from build123d import *

# Parameters (mm, degrees)
SKETCH1_R           = 3
SKETCH1_W           = 3.88
SKETCH1_H           = 3
BOSS_EXTRUDE1_DEPTH = 3
SKETCH2_R           = 1.0009
CUT_EXTRUDE1_DEPTH  = 516.692890771


with BuildPart() as part:
    # Sketch1 → Boss-Extrude1 (new body)
    with BuildSketch(Plane.XY):
        Polygon((-398.2841, 298.0765), (-386.271234014, 299.794262601), (-329.587365996, 299.794262601), (-329.587365996, 281.358737399), (-386.271234014, 281.358737399), (-398.2841, 283.0765), (-419.587365996, 283.0765), (-419.587365996, 298.0765), align=None)
        with Locations((-404.586054436, 290.5765)):
            Circle(SKETCH1_R, mode=Mode.SUBTRACT)
        with Locations((-369.044562351, 293.935134885)):
            Rectangle(SKETCH1_W, SKETCH1_H, mode=Mode.SUBTRACT)
        with Locations((-369.044562351, 285.640934885)):
            Rectangle(SKETCH1_W, SKETCH1_H, mode=Mode.SUBTRACT)
        with Locations((-341.542562351, 293.935134885)):
            Rectangle(SKETCH1_W, SKETCH1_H, mode=Mode.SUBTRACT)
        with Locations((-341.542562351, 285.640934885)):
            Rectangle(SKETCH1_W, SKETCH1_H, mode=Mode.SUBTRACT)
    extrude(amount=BOSS_EXTRUDE1_DEPTH)

    # Sketch2 → Cut-Extrude1 (cut, through all)
    with BuildSketch(Plane.XY.offset(3)):
        with Locations((-414.786054436, 290.5765)):
            Circle(SKETCH2_R)
        with Locations((-410.936054436, 290.5765)):
            Circle(SKETCH2_R)
        with Locations((-398.236054436, 290.5765)):
            Circle(SKETCH2_R)
        with Locations((-394.386054436, 290.5765)):
            Circle(SKETCH2_R)
    extrude(amount=-CUT_EXTRUDE1_DEPTH, mode=Mode.SUBTRACT)


solid = part.part
Design review of the part built by this model. Coordinates are the model's own, in mm. A direction names the side the tool comes from. Round coordinates to 2 decimals unless told otherwise and drop trailing zeros. Order: outer loops, then holes, each group sorted by start corner. A loop starts at its lowest first (then second) coordinate and runs counter-clockwise, first axis right, second up.
1) For L1, parallel to Y at x = -340.5, z = 2.4; L2, parallel to X at y = 290.5, z = 2.75; L3, parallel to X at y = 285.5, z = 0.7, list the stretches that pass through material, from the lowest coordinate up.
The answers:
L1: y = 281.36 to 284.14, 287.14 to 292.44, 295.44 to 299.79
L2: x = -419.59 to -415.78, -413.79 to -411.93, -409.94 to -407.59, -401.59 to -399.23, -397.24 to -395.38, -393.39 to -329.59
L3: x = -419.59 to -370.98, -367.1 to -343.48, -339.6 to -329.59
2) Draft analysis for pull direction X (two halves, no side actions). For faces 4 (the flat face through (-329.587, 291, 1)), 5 (the flat face through (-370.985, 294, 1)), 6 (the flat face through (-392.194, 282.206, 1.479)), 7 (the flat face through (-374, 291, 3)), state which applies: released by +X, released by -X, zero draft, split by the parting line, or undercut.
The answers:
face 4: released by +X
face 5: undercut
face 6: released by -X
face 7: zero draft
3) Consider section A-A (y = 286). State the section outline as (x, z) points.
The answers:
outline: (-419.59, 0) - (-370.98, 0) - (-370.98, 3) - (-419.59, 3) - close; (-367.1, 0) - (-343.48, 0) - (-343.48, 3) - (-367.1, 3) - close; (-339.6, 0) - (-329.59, 0) - (-329.59, 3) - (-339.6, 3) - close
4) Consider section B-B (z = 1.4). Count the separate pieces of the cut face and the enclosed holes in it, plus the area to 3 significant figures.
The answers:
separate pieces: 1
enclosed holes: 9
area: 1,480 mm2
5) Machinability: for faces 1 (the flat face through (-409, 283.076, 1)), 2 (the flat face through (-358, 299.794, 1)), 3 (the flat face through (-342, 287.141, 1)), which of the approach directions +Z, -Z, +X, -X, +Y, -Y give a long, thin tool a straight path to every point of the face, cutting with its end or side? Answer none if there is none.
The answers:
face 1: +Z, -Z, -X, -Y
face 2: +Z, -Z, +X, -X, +Y
face 3: +Z, -Z
6) Consider section C-C (x = -392.5). State the section outline as (y, z) points, plus the area to 3 significant figures.
The answers:
outline: (282.25, 0) - (298.9, 0) - (298.9, 3) - (282.25, 3) - close
area: 50.0 mm2
7) Clearance check with a flat-ended pin moving along its axis: pin 1 Ø1.5 at (x, z) = (-412, 1) entering from -Y. State where the tip first meets the part, or that it passes through.
The answers:
pin 1: stops at y = 283.08
